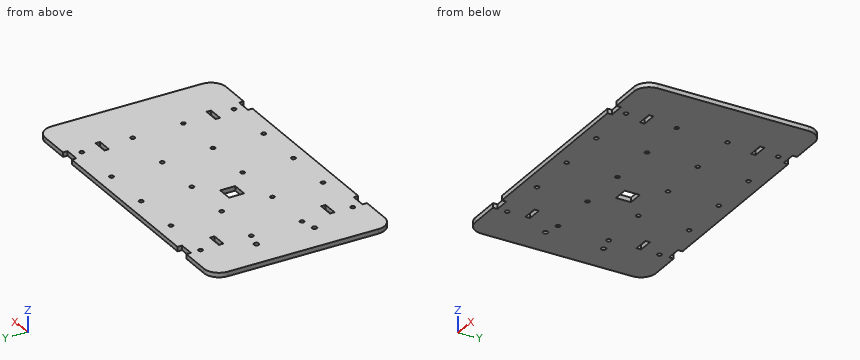
Autodesk Inventor part; units mm, degrees
ref_plane "Work Plane1" through (0, 60, 0) normal (0, 1, 0) x (1, 0, 0)
ref_plane "Work Plane66" through (0, 60, 0) normal (0, 1, 0) x (1, 0, 0)
ref_plane "Work Plane67" through (100, 0, 0) normal (-1, 0, 0) x (0, 0, 1)
sketch "Sketch1" plane through (0, 0, 0) normal (0, 0, 1) x (1, 0, 0)
  line L0 (0, 0) -> (200, 0)
  line L1 (200, 0) -> (200, 120)
  line L2 (200, 120) -> (0, 120)
  line L3 (0, 120) -> (0, 0)
  dimension "d6" = 200
  dimension "d7" = 120
extrude "Extrusion1" add sketch "Sketch1" along normal blind 3
sketch "Sketch2" plane through (0, 0, 3) normal (0, 0, 1) x (1, 0, 0)
  line L0 (0, 120) -> (0, 0) construction
  line L1 (0, 60) -> (200, 60) construction
  line L2 (200, 0) -> (200, 120) construction
  line L3 (200, 120) -> (0, 120) construction
  line L4 (100, 120) -> (100, 0) construction
  line L5 (0, 0) -> (200, 0) construction
  point P0 (30, 43.15)
  dimension "d10" = 16.85
  dimension "d11" = 30
hole "Hole1" at (30, 43.15, 3) direction (0, 0, -1) diameter 2.85 end through all
ref_plane "Work Plane1" through (0, 60, 0) normal (0, 1, 0) x (1, 0, 0)
mirror "Mirror1" about plane through (0, 60, 0) normal (0, 1, 0) of "Hole1"
pattern_linear "Rectangular Pattern1" count 2 spacing 33.7 along (1, 0, 0) of "Hole1", "Mirror1"
pattern_linear "Rectangular Pattern2" count 4 spacing 33.7 along (1, 0, 0) count 2 spacing 33.7 along (0, 1, 0) of "Hole1", "Mirror1", "Rectangular Pattern1"
mirror "Mirror2" about plane through (0, 60, 0) normal (0, 1, 0) of "Hole1", "Mirror1", "Rectangular Pattern1", "Rectangular Pattern2"
sketch "Sketch3" plane through (0, 0, 3) normal (0, 0, 1) x (1, 0, 0)
  line L0 (75.55, 65) -> (85.55, 65)
  line L1 (85.55, 65) -> (85.55, 55)
  line L2 (85.55, 55) -> (75.55, 55)
  line L3 (75.55, 55) -> (75.55, 65)
  circle A0 centre (63.7, 76.85) radius 1.425 construction
  circle A1 centre (97.4, 43.15) radius 1.425 construction
  line L4 (63.7, 76.85) -> (97.4, 43.15) construction
  circle A2 centre (97.4, 76.85) radius 1.425 construction
  circle A3 centre (63.7, 43.15) radius 1.425 construction
  line L5 (63.7, 43.15) -> (97.4, 76.85) construction
  point P0 (0, 0)
  point P1 (80.55, 65)
  point P2 (80.55, 60)
  point P3 (85.55, 60)
  point P4 (80.55, 60)
  dimension "d28" = 10
  dimension "d29" = 10
extrude "Extrusion2" cut sketch "Sketch3" against normal through all
sketch "Sketch4" plane through (0, 0, 3) normal (0, 0, 1) x (1, 0, 0)
  line L0 (0, 0) -> (200, 0) construction
  line L1 (30, 0) -> (40, 0)
  line L2 (40, 0) -> (40, 3)
  line L3 (40, 3) -> (30, 3)
  line L4 (30, 3) -> (30, 0)
  line L5 (0, 120) -> (0, 0) construction
  line L6 (30, 24.6) -> (40, 24.6)
  line L7 (40, 24.6) -> (40, 21.6)
  line L8 (40, 21.6) -> (30, 21.6)
  line L9 (30, 21.6) -> (30, 24.6)
  dimension "d32" = 3
  dimension "d33" = 10
  dimension "d34" = 30
  dimension "d35" = 18.6
  dimension "d36" = 3
  dimension "d37" = 10
extrude "Extrusion3" cut sketch "Sketch4" against normal through all
ref_plane "Work Plane66" through (0, 60, 0) normal (0, 1, 0) x (1, 0, 0)
mirror "Mirror3" about plane through (0, 60, 0) normal (0, 1, 0) of "Extrusion3"
ref_plane "Work Plane67" through (100, 0, 0) normal (-1, 0, 0) x (0, 0, 1)
mirror "Mirror4" about plane through (100, 0, 0) normal (-1, 0, 0) of "Extrusion3", "Mirror3"
sketch "Sketch5" plane through (0, 0, 3) normal (0, 0, 1) x (1, 0, 0)
  line L0 (0, 120) -> (0, 0) construction
  line L1 (0, 120) -> (0, 0) construction
  line L2 (0, 60) -> (200, 60) construction
  line L3 (200, 0) -> (200, 120) construction
  point P0 (20, 40.7)
  dimension "d40" = 20
  dimension "d41" = 19.3
hole "Hole2" at (20, 40.7, 3) direction (0, 0, -1) diameter 3.242 end through all
ref_plane "Work Plane68" through (40, 60, 0) normal (0, -1, 0) x (1, 0, 0)
mirror "Mirror5" about plane through (40, 60, 0) normal (0, -1, 0) of "Hole2"
fillet "Fillet1" radius 10 4 edges at (0, 120, 1.5) (0, 0, 1.5) (200, 0, 1.5) (200, 120, 1.5)
ref_plane "Work Plane2" through (0, 60, 0) normal (0, 1, 0) x (1, 0, 0)
ref_plane "Work Plane4" through (33.7, 60, 0) normal (0, 1, 0) x (1, 0, 0)
ref_plane "Work Plane5" through (33.7, 60, 0) normal (0, 1, 0) x (1, 0, 0)
ref_plane "Work Plane6" through (33.7, 60, 0) normal (0, 1, 0) x (1, 0, 0)
ref_plane "Work Plane7" through (67.4, 60, 0) normal (0, 1, 0) x (1, 0, 0)
ref_plane "Work Plane8" through (101.1, 60, 0) normal (0, 1, 0) x (1, 0, 0)
ref_plane "Work Plane9" through (0, 93.7, 0) normal (0, 1, 0) x (1, 0, 0)
ref_plane "Work Plane10" through (33.7, 93.7, 0) normal (0, 1, 0) x (1, 0, 0)
ref_plane "Work Plane11" through (67.4, 93.7, 0) normal (0, 1, 0) x (1, 0, 0)
ref_plane "Work Plane12" through (101.1, 93.7, 0) normal (0, 1, 0) x (1, 0, 0)
ref_plane "Work Plane13" through (33.7, 60, 0) normal (0, 1, 0) x (1, 0, 0)
ref_plane "Work Plane14" through (67.4, 60, 0) normal (0, 1, 0) x (1, 0, 0)
ref_plane "Work Plane15" through (101.1, 60, 0) normal (0, 1, 0) x (1, 0, 0)
ref_plane "Work Plane16" through (0, 93.7, 0) normal (0, 1, 0) x (1, 0, 0)
ref_plane "Work Plane17" through (33.7, 93.7, 0) normal (0, 1, 0) x (1, 0, 0)
ref_plane "Work Plane18" through (67.4, 93.7, 0) normal (0, 1, 0) x (1, 0, 0)
ref_plane "Work Plane19" through (101.1, 93.7, 0) normal (0, 1, 0) x (1, 0, 0)
ref_plane "Work Plane20" through (67.4, 60, 0) normal (0, 1, 0) x (1, 0, 0)
ref_plane "Work Plane21" through (101.1, 60, 0) normal (0, 1, 0) x (1, 0, 0)
ref_plane "Work Plane22" through (134.8, 60, 0) normal (0, 1, 0) x (1, 0, 0)
ref_plane "Work Plane23" through (33.7, 93.7, 0) normal (0, 1, 0) x (1, 0, 0)
ref_plane "Work Plane24" through (67.4, 93.7, 0) normal (0, 1, 0) x (1, 0, 0)
ref_plane "Work Plane25" through (101.1, 93.7, 0) normal (0, 1, 0) x (1, 0, 0)
ref_plane "Work Plane26" through (134.8, 93.7, 0) normal (0, 1, 0) x (1, 0, 0)
ref_plane "Work Plane27" through (67.4, 60, 0) normal (0, 1, 0) x (1, 0, 0)
ref_plane "Work Plane28" through (101.1, 60, 0) normal (0, 1, 0) x (1, 0, 0)
ref_plane "Work Plane29" through (134.8, 60, 0) normal (0, 1, 0) x (1, 0, 0)
ref_plane "Work Plane30" through (33.7, 93.7, 0) normal (0, 1, 0) x (1, 0, 0)
ref_plane "Work Plane31" through (67.4, 93.7, 0) normal (0, 1, 0) x (1, 0, 0)
ref_plane "Work Plane32" through (101.1, 93.7, 0) normal (0, 1, 0) x (1, 0, 0)
ref_plane "Work Plane33" through (134.8, 93.7, 0) normal (0, 1, 0) x (1, 0, 0)
ref_plane "Work Plane34" through (0, 60, 0) normal (0, 1, 0) x (1, 0, 0)
ref_plane "Work Plane35" through (0, 60, 0) normal (0, 1, 0) x (1, 0, 0)
ref_plane "Work Plane36" through (33.7, 60, 0) normal (0, 1, 0) x (1, 0, 0)
ref_plane "Work Plane37" through (33.7, 60, 0) normal (0, 1, 0) x (1, 0, 0)
ref_plane "Work Plane38" through (134.8, 26.3, 0) normal (0, 1, 0) x (1, 0, 0)
ref_plane "Work Plane39" through (101.1, 26.3, 0) normal (0, 1, 0) x (1, 0, 0)
ref_plane "Work Plane40" through (67.4, 26.3, 0) normal (0, 1, 0) x (1, 0, 0)
ref_plane "Work Plane41" through (33.7, 26.3, 0) normal (0, 1, 0) x (1, 0, 0)
ref_plane "Work Plane42" through (134.8, 60, 0) normal (0, 1, 0) x (1, 0, 0)
ref_plane "Work Plane43" through (101.1, 60, 0) normal (0, 1, 0) x (1, 0, 0)
ref_plane "Work Plane44" through (67.4, 60, 0) normal (0, 1, 0) x (1, 0, 0)
ref_plane "Work Plane45" through (134.8, 26.3, 0) normal (0, 1, 0) x (1, 0, 0)
ref_plane "Work Plane46" through (101.1, 26.3, 0) normal (0, 1, 0) x (1, 0, 0)
ref_plane "Work Plane47" through (67.4, 26.3, 0) normal (0, 1, 0) x (1, 0, 0)
ref_plane "Work Plane48" through (33.7, 26.3, 0) normal (0, 1, 0) x (1, 0, 0)
ref_plane "Work Plane49" through (134.8, 60, 0) normal (0, 1, 0) x (1, 0, 0)
ref_plane "Work Plane50" through (101.1, 60, 0) normal (0, 1, 0) x (1, 0, 0)
ref_plane "Work Plane51" through (67.4, 60, 0) normal (0, 1, 0) x (1, 0, 0)
ref_plane "Work Plane52" through (101.1, 26.3, 0) normal (0, 1, 0) x (1, 0, 0)
ref_plane "Work Plane53" through (67.4, 26.3, 0) normal (0, 1, 0) x (1, 0, 0)
ref_plane "Work Plane54" through (33.7, 26.3, 0) normal (0, 1, 0) x (1, 0, 0)
ref_plane "Work Plane55" through (0, 26.3, 0) normal (0, 1, 0) x (1, 0, 0)
ref_plane "Work Plane56" through (101.1, 60, 0) normal (0, 1, 0) x (1, 0, 0)
ref_plane "Work Plane57" through (67.4, 60, 0) normal (0, 1, 0) x (1, 0, 0)
ref_plane "Work Plane58" through (33.7, 60, 0) normal (0, 1, 0) x (1, 0, 0)
ref_plane "Work Plane59" through (101.1, 26.3, 0) normal (0, 1, 0) x (1, 0, 0)
ref_plane "Work Plane60" through (67.4, 26.3, 0) normal (0, 1, 0) x (1, 0, 0)
ref_plane "Work Plane61" through (33.7, 26.3, 0) normal (0, 1, 0) x (1, 0, 0)
ref_plane "Work Plane62" through (0, 26.3, 0) normal (0, 1, 0) x (1, 0, 0)
ref_plane "Work Plane63" through (101.1, 60, 0) normal (0, 1, 0) x (1, 0, 0)
ref_plane "Work Plane64" through (67.4, 60, 0) normal (0, 1, 0) x (1, 0, 0)
ref_plane "Work Plane65" through (33.7, 60, 0) normal (0, 1, 0) x (1, 0, 0)
equation "\"d36\" = d32"
equation "\"d37\" = d33"
properties part number "FPVchasisdraft2"
Source: CAD feature listing. Evaluate the final solid. Frame: model axes, mm. Round coordinates to 2 decimals unless told otherwise and drop trailing zeros.
(1) Material intervals for probe 1 along X at (y, z) = (9.45, 1.1) (3 decimals); probe 2 along Y at (x, z) = (32, 1.75); probe 3 along Y at (x, z) = (20, 1.2), sorted ascending.
From the geometry:
probe 1: x = 0.015 to 28.575, 31.425 to 62.275, 65.125 to 95.975, 98.825 to 129.675, 132.525 to 163.375, 166.225 to 199.985
probe 2: y = 3 to 21.6, 24.6 to 95.4, 98.4 to 117
probe 3: y = 0 to 39.08, 42.32 to 77.68, 80.92 to 120
(2) Contact query for flat-ended pins moving along their axis: pin 1 Ø1.5 at (x, z) = (36, 1.5) entering from +Y; pin 2 Ø0.9 at (y, z) = (119, 1.5) entering from -X; pin 3 Ø1.7 at (x, y) = (131.1, 43.15) entering from +Z. Output: stop coordinate, or through.
From the geometry:
pin 1: stops at y = 117
pin 2: stops at x = 4.81
pin 3: passes through
(3) Section query A-A (z = 1.1). Give the number of separate pieces and of enclosed holes in the cut face, and give its area (3 significant figures).
From the geometry:
separate pieces: 1
enclosed holes: 27
area: 23,400 mm2
